CAD build for the part. Positions are in the model's coordinates, mm. Coordinates: 2 decimals unless noted, no trailing zeros. Loops run counter-clockwise (first coordinate to the right, second up) from the corner with the lowest first, then second, coordinate; pieces in that order, holes last. Notation, with made-up numbers: (29.25, -31) -> (50.25, -31) arc R20 ccw to (50.25, -7) -> close; hole circle Ø2 at (-24, 12.5). An arc over 180 degrees is marked (long way). Return JSON: item names as keys, results as strings. Group by question number.
(1) Flat gauge pins, fed straight in: pin 1 Ø6 at (y, z) = (-15.5, 2) entering from +X; pin 2 Ø1.5 at (x, z) = (14, 11) entering from +Y; pin 3 Ø1.5 at (y, z) = (5.5, 7.5) entering from +X. Where does each tip first touch, or does it go through?
(2) Saw through at C-C on z = 1. Write the cut outline in (x, y) (3 decimals).
(3) Saw through at B-B on x = -14.5. Write the cut outline in (y, z), then the cut area to 3 significant figures.
(4) Saw through at A-A on y = -7.5. Write the cut outline in (x, z), then the cut area to 3 significant figures.
(5) Probe L1, parallel to Y at x = 0.5, z = 1.25; L2, parallel to X at y = -22.5, z = 14.75 (3 decimals); L3, parallel to Y at x = 23, z = 12.25. List the from-to ranges inside material, lowest first.
```python
from build123d import *

# Parameters (mm, degrees)
F1_DEPTH = 16


with BuildPart() as f1:
    # F0 (on Top) → F1 (new body)
    with BuildSketch(Plane.XY):
        with BuildLine():
            ThreePointArc((-23.069359, 23.069359), (-30.14157, 12.485047), (-32.625, 0))
            ThreePointArc((-32.625, 0), (-12.485047, -30.14157), (23.069359, -23.069359))
            ThreePointArc((23.069359, -23.069359), (30.14157, -12.485047), (32.625, 0))
            ThreePointArc((32.625, 0), (12.485047, 30.14157), (-23.069359, 23.069359))
        make_face()
        with BuildLine():
            ThreePointArc((-22.645095, 22.645095), (12.255437, 29.587242), (32.025, 0))
            ThreePointArc((32.025, 0), (29.587242, -12.255437), (22.645095, -22.645095))
            ThreePointArc((22.645095, -22.645095), (-12.255437, -29.587242), (-32.025, 0))
            ThreePointArc((-32.025, 0), (-29.587242, 12.255437), (-22.645095, 22.645095))
        make_face(mode=Mode.SUBTRACT)
    extrude(amount=F1_DEPTH)


solid = f1.part
```
Geometry results:
{
 "1": {"pin 1": "x = 30.14", "pin 2": "y = 29.81", "pin 3": "x = 32.28"},
 "2": {"outline": "circle Ø65.25 at (0, 0); hole (-32.025, 0) arc R32.025 ccw to (22.645, -22.645) arc R32.025 ccw to (32.025, 0) arc R32.025 ccw to (-22.645, 22.645) arc R32.025 ccw to start"},
 "3": {"outline": "(-29.23, 0) -> (-28.55, 0) -> (-28.55, 16) -> (-29.23, 16) -> close; (28.55, 0) -> (29.23, 0) -> (29.23, 16) -> (28.55, 16) -> close", "area": "21.5 mm²"},
 "4": {"outline": "(-31.75, 0) -> (-31.13, 0) -> (-31.13, 16) -> (-31.75, 16) -> close; (31.13, 0) -> (31.75, 0) -> (31.75, 16) -> (31.13, 16) -> close", "area": "19.7 mm²"},
 "5": {"L1": "-32.62 to -32.02, 32.02 to 32.62", "L2": "-23.625 to -22.789, 22.789 to 23.625", "L3": "-23.14 to -22.28, 22.28 to 23.14"}
}
